from build123d import *

# Parameters (mm, degrees)
BOSS_EXTRUDE3_DEPTH   = 10
BOSS_EXTRUDE3_2_DEPTH = 10
BOSS_EXTRUDE3_3_DEPTH = 10
BOSS_EXTRUDE3_4_DEPTH = 10
BOSS_EXTRUDE4_DEPTH   = 7


with BuildPart() as part:
    # Sketch1 → Boss-Extrude3 (new body)
    with BuildSketch(Plane(origin=(0, 0, 0), x_dir=(1, 0, 0), z_dir=(0, 1, 0))):
        Polygon((-12.139188815, -6.424573702), (-15.139188815, -8.156624509), (-8.139188815, -12.198076394), (-8.139188815, -20.280980162), (-15.139188815, -24.322432047), (-12.139188815, -26.054482854), (-5.139188815, -22.01303097), (-5.139188815, -10.466025586), align=None)
    extrude(amount=BOSS_EXTRUDE3_DEPTH)



with BuildPart() as body_2:
    # Sketch1 → Boss-Extrude3 2 (new body)
    with BuildSketch(Plane(origin=(0, 0, 0), x_dir=(1, 0, 0), z_dir=(0, 1, 0))):
        Polygon((7.860811185, -6.424573702), (4.860811185, -8.156624509), (11.860811185, -12.198076394), (11.860811185, -20.280980162), (4.860811185, -24.322432047), (7.860811185, -26.054482854), (14.860811185, -22.01303097), (14.860811185, -10.466025586), align=None)
    extrude(amount=BOSS_EXTRUDE3_2_DEPTH)


with BuildPart() as body_3:
    # Sketch1 → Boss-Extrude3 3 (new body)
    with BuildSketch(Plane(origin=(0, 0, 0), x_dir=(1, 0, 0), z_dir=(0, 1, 0))):
        Polygon((34.860811185, -10.466025586), (27.860811185, -6.424573702), (24.860811185, -8.156624509), (31.860811185, -12.198076394), (31.860811185, -20.280980162), (24.860811185, -24.322432047), (27.860811185, -26.054482854), (34.860811185, -22.01303097), align=None)
    extrude(amount=BOSS_EXTRUDE3_3_DEPTH)


with BuildPart() as body_4:
    # Sketch1 → Boss-Extrude3 4 (new body)
    with BuildSketch(Plane(origin=(0, 0, 0), x_dir=(1, 0, 0), z_dir=(0, 1, 0))):
        Polygon((54.860811185, -22.01303097), (54.860811185, -10.466025586), (47.860811185, -6.424573702), (44.860811185, -8.156624509), (51.860811185, -12.198076394), (51.860811185, -20.280980162), (44.860811185, -24.322432047), (47.860811185, -26.054482854), align=None)
    extrude(amount=BOSS_EXTRUDE3_4_DEPTH)


with BuildPart() as part_1:
    add(part.part)

    add(body_2.part)  # Boss-Extrude4 merges body 2

    add(body_3.part)  # Boss-Extrude4 merges body 3

    add(body_4.part)  # Boss-Extrude4 merges body 4
    # Sketch1_8 → Boss-Extrude4 (add)
    with BuildSketch(Plane(origin=(0, 0, 0), x_dir=(1, 0, 0), z_dir=(0, 1, 0))):
        Polygon((-12.139188815, -26.054482854), (-15.139188815, -24.322432047), (-18.139188815, -26.054482854), (-15.139188815, -27.786533662), align=None)
        Polygon((-15.139188815, -8.156624509), (-18.139188815, -6.424573702), (-25.139188815, -10.466025586), (-25.139188815, -22.01303097), (-18.139188815, -26.054482854), (-15.139188815, -24.322432047), (-22.139188815, -20.280980162), (-22.139188815, -12.198076394), align=None)
        Polygon((-15.139188815, -4.692522894), (-18.139188815, -6.424573702), (-15.139188815, -8.156624509), (-12.139188815, -6.424573702), align=None)
        Polygon((4.860811185, -4.692522894), (1.860811185, -6.424573702), (4.860811185, -8.156624509), (7.860811185, -6.424573702), align=None)
        Polygon((4.860811185, -8.156624509), (1.860811185, -6.424573702), (-5.139188815, -10.466025586), (-5.139188815, -22.01303097), (1.860811185, -26.054482854), (4.860811185, -24.322432047), (-2.139188815, -20.280980162), (-2.139188815, -12.198076394), align=None)
        Polygon((7.860811185, -26.054482854), (4.860811185, -24.322432047), (1.860811185, -26.054482854), (4.860811185, -27.786533662), align=None)
        Polygon((27.860811185, -26.054482854), (24.860811185, -24.322432047), (21.860811185, -26.054482854), (24.860811185, -27.786533662), align=None)
        Polygon((17.860811185, -12.198076394), (24.860811185, -8.156624509), (21.860811185, -6.424573702), (14.860811185, -10.466025586), (14.860811185, -22.01303097), (21.860811185, -26.054482854), (24.860811185, -24.322432047), (17.860811185, -20.280980162), align=None)
        Polygon((24.860811185, -8.156624509), (27.860811185, -6.424573702), (24.860811185, -4.692522894), (21.860811185, -6.424573702), align=None)
        Polygon((44.860811185, -8.156624509), (47.860811185, -6.424573702), (44.860811185, -4.692522894), (41.860811185, -6.424573702), align=None)
        Polygon((37.860811185, -12.198076394), (44.860811185, -8.156624509), (41.860811185, -6.424573702), (34.860811185, -10.466025586), (34.860811185, -22.01303097), (41.860811185, -26.054482854), (44.860811185, -24.322432047), (37.860811185, -20.280980162), align=None)
        Polygon((44.860811185, -27.786533662), (47.860811185, -26.054482854), (44.860811185, -24.322432047), (41.860811185, -26.054482854), align=None)
    extrude(amount=BOSS_EXTRUDE4_DEPTH)


solid = part_1.part
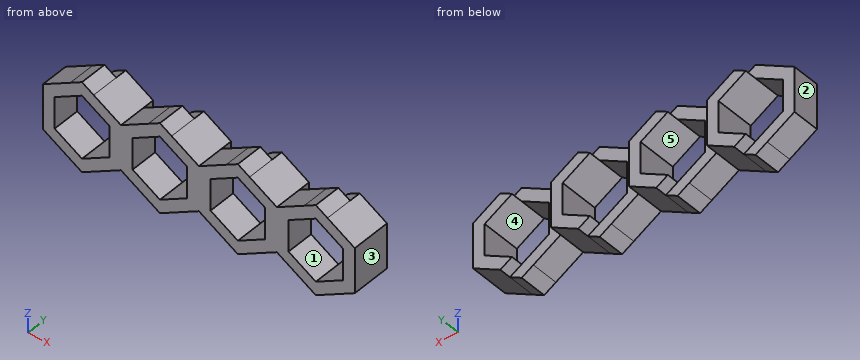
Build history of the part. All positions in model axes, mm. Face numbers are marked on the shaded views. A direction names the side the tool comes from. Coordinates: 2 decimals unless noted, no trailing zeros. Write each loop counter-clockwise with the first axis right and the second up, starting at its lowest first coordinate (ties: lowest second). Pieces come first, ordered by that corner, then holes.
(1) Mould opens along Z. For the marked faces 3, 4 and 5 say: pulls with the +Z half, pulls with the -Z half, needs draft (parallel to the pull), parting line crosses it, or undercut.
(2) Cut at D-D on x = 49. List the corners of the cut face in (y, z).
(3) Drill centre lines: line 1 (X direction, y = 3.75, z = 20.25); line 2 (X direction, y = 4.25, z = 7); line 3 (X direction, y = 7.25, z = 25.5). Where is each one in solid material? Low to high.
(4) Cut at A-A on z = 14. List the corners of the cut face in (x, y).
(5) Cut at C-C on z = 7.25. List the corners of the cut face in (x, y), and give its area (3 significant figures).
(6) Cut at B-B on y = 8. State how many separate pieces and enclosed holes the cut face has, and give its area (3 significant figures).
(7) Pin check, flat tips, straight feed: pin 1 Ø4 at (x, z) = (1.5, 18.5) entering from +Y; pin 2 Ø3 at (x, y) = (7.5, 4) entering from -Z; pin 3 Ø3 at (x, y) = (-2.5, 1.5) entering from -Z; pin 4 Ø1.5 at (x, y) = (-7.5, 3) entering from -Z. Stop position of each tip, or through.
(8) 3-axis set-ups, long thin cutter, end or side, ignore diameter. For the marked faces 1 and 2: which of +Z, -Z, +X, -X, +Y, -Y reach the whole face in a straight line?
Working result:
1. face 3: needs draft
1. face 4: undercut
1. face 5: undercut
2. outline: (0, 7.08) - (10, 7.08) - (10, 10.55) - (0, 10.55) - close; (0, 21.93) - (10, 21.93) - (10, 25.4) - (0, 25.4) - close
3. line 1: x = -25.14 to -22.14, -8.14 to -2.14, 11.86 to 17.86, 31.86 to 37.86, 51.86 to 54.86
3. line 2: x = -19.14 to -11.14, 0.86 to 8.86, 20.86 to 28.86, 40.86 to 48.86
3. line 3: x = -13.1 to -11.18, 6.9 to 8.82, 26.9 to 28.82, 46.9 to 48.82
4. outline: (-25.14, 0) - (-22.14, 0) - (-22.14, 7) - (-25.14, 7) - close; (-8.14, 0) - (-2.14, 0) - (-2.14, 7) - (-5.14, 7) - (-5.14, 10) - (-8.14, 10) - close; (11.86, 0) - (17.86, 0) - (17.86, 7) - (14.86, 7) - (14.86, 10) - (11.86, 10) - close; (31.86, 0) - (37.86, 0) - (37.86, 7) - (34.86, 7) - (34.86, 10) - (31.86, 10) - close; (51.86, 0) - (54.86, 0) - (54.86, 10) - (51.86, 10) - close
5. outline: (-19.57, 0) - (-10.71, 0) - (-10.71, 10) - (-13.57, 10) - (-13.57, 7) - (-19.57, 7) - close; (0.43, 0) - (9.29, 0) - (9.29, 10) - (6.43, 10) - (6.43, 7) - (0.43, 7) - close; (20.43, 0) - (29.29, 0) - (29.29, 10) - (26.43, 10) - (26.43, 7) - (20.43, 7) - close; (40.43, 0) - (49.29, 0) - (49.29, 10) - (46.43, 10) - (46.43, 7) - (40.43, 7) - close
5. area: 282 mm2
6. separate pieces: 4
6. enclosed holes: 0
6. area: 312 mm2
7. pin 1: passes through
7. pin 2: stops at z = 5.35
7. pin 3: stops at z = 8.08
7. pin 4: stops at z = 8.67
8. face 1: +Y, -Y
8. face 2: +Z, -Z, -X, +Y, -Y
